The listing builds one solid part. Answer for the finished solid, in the listing's coordinates (mm). A direction names the side the tool comes from. Give positions to 0.01 mm unless a question says otherwise; leave off trailing zeros. Order: outer loops, then holes, each group sorted by start corner. A loop starts at its lowest first (then second) coordinate and runs counter-clockwise, first axis right, second up.
```python
from build123d import *

# Parameters (mm, degrees)
CROQUIS1_W                 = 1
CROQUIS1_H                 = 7.62
SALIENTE_EXTRUIR1_START    = -3.81
SALIENTE_EXTRUIR1_DEPTH    = 2
MATRIZC1_COUNT             = 4
CORTAR_EXTRUIR1_DEPTH      = 27.019148718
CORTAR_EXTRUIR1_DEPTH_BACK = 27.019148718
CROQUIS4_W                 = 20.5
CROQUIS4_H                 = 3.56


with BuildPart() as part:
    # Croquis1 → Revolución1 (revolve)
    with BuildSketch(Plane.XY, mode=Mode.PRIVATE) as revoluci_n1_sk:
        with Locations((14.6, 0)):
            Rectangle(CROQUIS1_W, CROQUIS1_H)
    revolve(revoluci_n1_sk.sketch.rotate(Axis((0, 5.941666667, 0), (0, -1, 0)), 90), axis=Axis((0, 5.941666667, 0), (0, -1, 0)))

    # Croquis2 → Saliente-Extruir1 (add)
    with BuildSketch(Plane(origin=(0, 0, 0), x_dir=(1, 0, 0), z_dir=(0, 1, 0)).offset(SALIENTE_EXTRUIR1_START)):
        Polygon((8.5, -18.2), (-8.5, -18.2), (-8.5, -12.480384609), (-7.3, -12.480384609), (-7.3, -17.2), (7.3, -17.2), (7.3, -12.480384609), (8.5, -12.480384609), align=None)
    saliente_extruir1 = extrude(amount=SALIENTE_EXTRUIR1_DEPTH)

    # MatrizC1: Saliente-Extruir1 ×4 about axis
    matrizc1_axis = Axis((0, 0, 0), (0, 1, 0))
    for i in range(1, MATRIZC1_COUNT):
        add(saliente_extruir1.rotate(matrizc1_axis, i * 360 / MATRIZC1_COUNT))

    # Croquis4 → Cortar-Extruir1 (cut, two sides: drawn at the far end of the back side and taken through both)
    with BuildSketch(Plane.XY.offset(-CORTAR_EXTRUIR1_DEPTH_BACK)):
        with Locations((0, 2.03)):
            Rectangle(CROQUIS4_W, CROQUIS4_H)
    extrude(amount=CORTAR_EXTRUIR1_DEPTH + CORTAR_EXTRUIR1_DEPTH_BACK, mode=Mode.SUBTRACT)


solid = part.part
```
1) Find section A-A (y = 3). Write down the section's boundary in (x, z), then the cut area to 3 significant figures.
Geometry says:
outline: (-10.25, -11.09) - (-10.25, -9.68) arc R14.1 cw to (-10.25, 9.68) - (-10.25, 11.09) arc R15.1 ccw to start; (10.25, -11.09) arc R15.1 ccw to (10.25, 11.09) - (10.25, 9.68) arc R14.1 cw to (10.25, -9.68) - close
area: 46.3 mm2
2) A tool of negligible diameter and unlimited length cuts with its end or side. For faces 5 (the flat face through (15, -3, 8.5)), 6 (the flat face through (10.25, 2, 10)), 7 (the flat face through (0, -3, 18.2)), 8 (the flat face through (-15, -3, 7.3)), 9 (the flat face through (-18.2, -3, 0)), from which of +Z, -Z, +X, -X, +Y, -Y can it reach the whole face along a straight path? Write none if from no direction.
Geometry says:
face 5: +Z, +X, +Y, -Y
face 6: +Z, -Z, +Y
face 7: +Z, +X, -X, +Y, -Y
face 8: +Y, -Y
face 9: +Z, -Z, -X, +Y, -Y
3) Find section D-D (y = -2.75). Count the separate pieces of the cut face and the enclosed holes in it, then the cut area to 3 significant figures.
Geometry says:
separate pieces: 1
enclosed holes: 5
area: 201 mm2
4) Find section B-B (z = 0). Write down the section's boundary in (x, y), then the cut area to 3 significant figures.
Geometry says:
outline: (-18.2, -3.81) - (-17.2, -3.81) - (-17.2, -1.81) - (-18.2, -1.81) - close; (-15.1, -3.81) - (-14.1, -3.81) - (-14.1, 3.81) - (-15.1, 3.81) - close; (14.1, -3.81) - (15.1, -3.81) - (15.1, 3.81) - (14.1, 3.81) - close; (17.2, -3.81) - (18.2, -3.81) - (18.2, -1.81) - (17.2, -1.81) - close
area: 19.2 mm2
5) Given P1, Ø2, axis at x = 13, y = 0, coming from the -Z side; P2, Ø1.6, axis at y = -3, z = 16.5, coming from the +X side; P3, Ø0.6, axis at y = -3, z = 15, coming from the -X side, each flat-ended and moving along its own axis, determine where each tip first touches the part or whether it passes through.
Geometry says:
P1: stops at z = -9.17
P2: stops at x = 8.5
P3: stops at x = -8.5
6) Find section C-C (x = 0). Write down the section's boundary in (y, z).
Geometry says:
outline: (-3.81, -18.2) - (-1.81, -18.2) - (-1.81, -17.2) - (-3.81, -17.2) - close; (-3.81, -15.1) - (0.25, -15.1) - (0.25, -14.1) - (-3.81, -14.1) - close; (-3.81, 14.1) - (0.25, 14.1) - (0.25, 15.1) - (-3.81, 15.1) - close; (-3.81, 17.2) - (-1.81, 17.2) - (-1.81, 18.2) - (-3.81, 18.2) - close
7) Straight lines are drawn through the part: probe 1 along X at (y, z) = (-2, 0); probe 2 along X at (y, z) = (1.25, 0); probe 3 along X at (y, z) = (-2, -2.5). For each, find the intervals that lie inside material, in ascending order.
Geometry says:
probe 1: x = -18.2 to -17.2, -15.1 to -14.1, 14.1 to 15.1, 17.2 to 18.2
probe 2: x = -15.1 to -14.1, 14.1 to 15.1
probe 3: x = -18.2 to -17.2, -14.89 to -13.88, 13.88 to 14.89, 17.2 to 18.2
8) For a pull along X with two mould halves and no side action, classify faces 1 (the flat face through (-8.5, -3, 15)), 2 (the flat face through (-14.5, 3.81, 0.1)), 3 (the flat face through (18.2, -3, 0)), 4 (the flat face through (0, -3, 17.2)) as +X half, -X half, draft (parallel to the pull), parting line (faces both ways), or undercut.
Geometry says:
face 1: -X half
face 2: draft
face 3: +X half
face 4: undercut
